```python
from build123d import *

# Parameters (mm, degrees)
SKETCH_1_R      = 2.1
EXTRUDE_1_DEPTH = 5
EXTRUDE_START   = 5
SKETCH_1_3_W    = 6
SKETCH_1_3_H    = 12
EXTRUDE_2_DEPTH = 5
FILLET_2_R      = 3
EXTRUDE_3_DEPTH = 10


with BuildPart() as part:
    # 草图1 → 凸台-拉伸1 (new body)
    # profile 1 of 10: a face of its own
    with BuildSketch(Plane(origin=(0, 0, 0), x_dir=(1, 0, 0), z_dir=(0, 1, 0))):
        with BuildLine():
            Line((0, 22), (0, 0))
            Line((0, 0), (20, 0))
            Line((20, 0), (20, 22))
            Line((20, 22), (13, 22))
            Line((13, 22), (13, 17.968245837))
            ThreePointArc((13, 17.968245837), (13.862372436, 17.790569415), (14.25, 17))
            ThreePointArc((14.25, 17), (13.862372436, 16.209430585), (13, 16.031754163))
            Line((13, 16.031754163), (13, 10))
            Line((13, 10), (7, 10))
            Line((7, 10), (7, 16.031754163))
            ThreePointArc((7, 16.031754163), (5.75, 17), (7, 17.968245837))
            Line((7, 17.968245837), (7, 22))
            Line((7, 22), (0, 22))
        make_face()
        with Locations(Location((10, 4, 0), (0, 0, 270))):
            Circle(SKETCH_1_R, mode=Mode.SUBTRACT)
    # profile 2 of 10: a face of its own
    with BuildSketch(Plane(origin=(0, 0, 0), x_dir=(1, 0, 0), z_dir=(0, 1, 0))):
        with BuildLine():
            Line((13, 22), (7, 22))
            Line((7, 22), (7, 17.968245837))
            ThreePointArc((7, 17.968245837), (7.540569415, 17.612372436), (7.75, 17))
            ThreePointArc((7.75, 17), (7.540569415, 16.387627564), (7, 16.031754163))
            Line((7, 16.031754163), (7, 10))
            Line((7, 10), (13, 10))
            Line((13, 10), (13, 16.031754163))
            ThreePointArc((13, 16.031754163), (12.25, 17), (13, 17.968245837))
            Line((13, 17.968245837), (13, 22))
        make_face()
    # profile 3 of 10: a face of its own
    with BuildSketch(Plane(origin=(0, 0, 0), x_dir=(1, 0, 0), z_dir=(0, 1, 0))):
        with BuildLine():
            ThreePointArc((14.25, 17), (13.862372436, 17.790569415), (13, 17.968245837))
            Line((13, 17.968245837), (13, 16.031754163))
            ThreePointArc((13, 16.031754163), (13.862372436, 16.209430585), (14.25, 17))
        make_face()
    # profile 4 of 10: a face of its own
    with BuildSketch(Plane(origin=(0, 0, 0), x_dir=(1, 0, 0), z_dir=(0, 1, 0))):
        with BuildLine():
            Line((13, 16.031754163), (13, 17.968245837))
            ThreePointArc((13, 17.968245837), (12.25, 17), (13, 16.031754163))
        make_face()
    # profile 5 of 10: a face of its own
    with BuildSketch(Plane(origin=(0, 0, 0), x_dir=(1, 0, 0), z_dir=(0, 1, 0))):
        with BuildLine():
            ThreePointArc((14.25, 17), (13.862372436, 17.790569415), (13, 17.968245837))
            Line((13, 17.968245837), (13, 16.031754163))
            ThreePointArc((13, 16.031754163), (13.862372436, 16.209430585), (14.25, 17))
        make_face()
    # profile 6 of 10: a face of its own
    with BuildSketch(Plane(origin=(0, 0, 0), x_dir=(1, 0, 0), z_dir=(0, 1, 0))):
        with BuildLine():
            Line((13, 16.031754163), (13, 17.968245837))
            ThreePointArc((13, 17.968245837), (12.25, 17), (13, 16.031754163))
        make_face()
    # profile 7 of 10: a face of its own
    with BuildSketch(Plane(origin=(0, 0, 0), x_dir=(1, 0, 0), z_dir=(0, 1, 0))):
        with BuildLine():
            ThreePointArc((7.75, 17), (7.540569415, 17.612372436), (7, 17.968245837))
            Line((7, 17.968245837), (7, 16.031754163))
            ThreePointArc((7, 16.031754163), (7.540569415, 16.387627564), (7.75, 17))
        make_face()
    # profile 8 of 10: a face of its own
    with BuildSketch(Plane(origin=(0, 0, 0), x_dir=(1, 0, 0), z_dir=(0, 1, 0))):
        with BuildLine():
            Line((7, 16.031754163), (7, 17.968245837))
            ThreePointArc((7, 17.968245837), (5.75, 17), (7, 16.031754163))
        make_face()
    # profile 9 of 10: a face of its own
    with BuildSketch(Plane(origin=(0, 0, 0), x_dir=(1, 0, 0), z_dir=(0, 1, 0))):
        with BuildLine():
            ThreePointArc((7.75, 17), (7.540569415, 17.612372436), (7, 17.968245837))
            Line((7, 17.968245837), (7, 16.031754163))
            ThreePointArc((7, 16.031754163), (7.540569415, 16.387627564), (7.75, 17))
        make_face()
    # profile 10 of 10: a face of its own
    with BuildSketch(Plane(origin=(0, 0, 0), x_dir=(1, 0, 0), z_dir=(0, 1, 0))):
        with BuildLine():
            Line((7, 16.031754163), (7, 17.968245837))
            ThreePointArc((7, 17.968245837), (5.75, 17), (7, 16.031754163))
        make_face()
    extrude(amount=EXTRUDE_1_DEPTH)

    # 草图1<3> → 凸台-拉伸2 (add)
    with BuildSketch(Plane(origin=(0, 0, 0), x_dir=(1, 0, 0), z_dir=(0, 1, 0)).offset(EXTRUDE_START)):
        with Locations((10, 16)):
            Rectangle(SKETCH_1_3_W, SKETCH_1_3_H)
    extrude(amount=EXTRUDE_2_DEPTH)

    # 圆角2
    fillet_2_edges = [part.edges().sort_by_distance(p)[0] for p in [
        (20, 2.5, 0),
        (0, 2.5, 0),
        (0, 2.5, -22),
        (20, 2.5, -22),
    ]]
    fillet(fillet_2_edges, radius=FILLET_2_R)

    # 草图2 → 凸台-拉伸3 (add)
    with BuildSketch(Plane.XZ):
        with BuildLine():
            Line((3, -22), (17, -22))
            ThreePointArc((17, -22), (19.121320344, -21.121320344), (20, -19))
            Line((20, -19), (20, -14))
            Line((20, -14), (0, -14))
            Line((0, -14), (0, -19))
            ThreePointArc((0, -19), (0.878679656, -21.121320344), (3, -22))
        make_face()
    extrude(amount=EXTRUDE_3_DEPTH)


solid = part.part
```
The listing builds one solid part. Answer for the finished solid, in the listing's coordinates (mm). A direction names the side the tool comes from. Coordinates: 2 decimals unless noted, no trailing zeros. Order: outer loops, then holes, each group sorted by start corner. A loop starts at its lowest first (then second) coordinate and runs counter-clockwise, first axis right, second up. Notation, with made-up numbers: M -4,57.5 L 23,57.5 A18 cw 23,88.5 Z; hole C 4,-28 d8. An arc over 180 degrees is marked long. Answer as a JSON object with one key per item and string values. Group by question number.
1. A tool of negligible diameter and unlimited length cuts with its end or side. For faces 5 (the cylindrical face through (19.1, 2.54, -0.86)), 6 (the flat face through (7, 7, -16)), 7 (the flat face through (10, 0, -7)), 8 (the flat face through (10, 7, -10)), 9 (the flat face through (13, 7, -16)), from which of +Z, -Z, +X, -X, +Y, -Y can it reach the whole face along a straight path? Write none if from no direction.
2. Flat-ended cylindrical pins translate along their axes: P1, Ø1.5, axis at x = 12.5, z = -6, coming from the -Y side; P2, Ø1.5, axis at y = 7, z = -14, coming from the -X side. Find the tip coordinate at first contact, or state that the pin passes through.
3. Straight lines are drawn through the part: line 1 (X direction, y = 3.65, z = -4); line 2 (Y direction, x = 9.25, z = -1.5); line 3 (Z direction, x = 8.5, y = -1.5). For each, find the intervals that lie inside material, in ascending order.
4. Section A-A on x = 10 is taken. Write down the section's boundary in (y, z), then the cut area to 3 significant figures.
5. Section B-B on z = -16 is taken. Write down the section's boundary in (x, y).
6. Section D-D on y = 7.75 is taken. Write down the section's boundary in (x, z), then the cut area to 3 significant figures.
7. Section C-C on z = -4 is taken. Write down the section's boundary in (x, y), then the cut area to 3 significant figures.
8. Determine the mould class of faces 1 (the flat face through (10, 2, 0)), 2 (the flat face through (20, 1, -13)), 3 (the cylindrical face through (12.082, 2.465, -4.273)), 4 (the cylindrical face through (0.86, 2.54, -0.9)) for opening direction X: released by +X, released by -X, zero draft, split by the parting line, or undercut.
Values follow:
{
 "1": {"face 5": "+Z, +X, +Y, -Y", "face 6": "+Z, -Z, -X, +Y", "face 7": "+Z, +X, -X, -Y", "face 8": "+Z, +X, -X, +Y", "face 9": "+Z, -Z, +X, +Y"},
 "2": {"P1": "y = 0", "P2": "x = 7"},
 "3": {"line 1": "0 to 7.9, 12.1 to 20", "line 2": "0 to 5", "line 3": "-22 to -14"},
 "4": {"outline": "M -10,-22 L 10,-22 L 10,-10 L 5,-10 L 5,-6.1 L 0,-6.1 L 0,-14 L -10,-14 Z; M 0,-1.9 L 5,-1.9 L 5,0 L 0,0 Z", "area": "229 mm2"},
 "5": {"outline": "M 0,-10 L 20,-10 L 20,5 L 13,5 L 13,10 L 7,10 L 7,5 L 0,5 Z"},
 "6": {"outline": "M 7,-22 L 13,-22 L 13,-10 L 7,-10 Z", "area": "72.0 mm2"},
 "7": {"outline": "M 0,0 L 7.9,0 L 7.9,5 L 0,5 Z; M 12.1,0 L 20,0 L 20,5 L 12.1,5 Z", "area": "79.0 mm2"},
 "8": {"face 1": "zero draft", "face 2": "released by +X", "face 3": "undercut", "face 4": "released by -X"}
}
